Build history of the part. All positions in model axes, mm. Face numbers are marked on the shaded views. A direction names the side the tool comes from. Coordinates: 2 decimals unless noted, no trailing zeros. Order: outer loops, then holes, each group sorted by start corner. A loop starts at its lowest first (then second) coordinate and runs counter-clockwise, first axis right, second up. Notation, with made-up numbers: (9, 35) - (61, 35) arc R28 ccw to (61, 61) - close; hole circle Ø6 at (27.5, 33). An arc over 180 degrees is marked (long way). Return JSON: item names as keys, results as strings.
from build123d import *

# Parameters (mm, degrees)
EXTRUSION1_DEPTH = 70
EXTRUSION2_REACH = 3
ESQUISSE2_R      = 2
EXTRUSION3_REACH = 3
ESQUISSE3_R      = 2


with BuildPart() as part:
    # Esquisse1 → Extrusion1 (new body)
    with BuildSketch(Plane(origin=(0, 0, 0), x_dir=(1, 0, 0), z_dir=(0, 1, 0))):
        Polygon((0, 0), (0, 16), (1, 16), (1, 1), (16, 1), (16, 0), align=None)
    extrude(amount=EXTRUSION1_DEPTH)

    # Esquisse2 → Extrusion2 (cut, up to next)
    with BuildSketch(Plane(origin=(1, 0, 0), x_dir=(0, 0, -1), z_dir=(1, 0, 0)), mode=Mode.PRIVATE) as extrusion2_sk1:
        with Locations((8.5, 16.5)):
            Circle(ESQUISSE2_R)
    extrusion2_tool1 = extrude(extrusion2_sk1.sketch, amount=-EXTRUSION2_REACH, mode=Mode.PRIVATE) & part.part
    add(extrusion2_tool1.solids().sort_by_distance((1, 16.5, -8.5))[0], mode=Mode.SUBTRACT)
    # Esquisse2 → Extrusion2 (cut, up to next)
    with BuildSketch(Plane(origin=(1, 0, 0), x_dir=(0, 0, -1), z_dir=(1, 0, 0)), mode=Mode.PRIVATE) as extrusion2_sk2:
        with Locations((8.5, 6.5)):
            Circle(ESQUISSE2_R)
    extrusion2_tool2 = extrude(extrusion2_sk2.sketch, amount=-EXTRUSION2_REACH, mode=Mode.PRIVATE) & part.part
    add(extrusion2_tool2.solids().sort_by_distance((1, 6.5, -8.5))[0], mode=Mode.SUBTRACT)
    # Esquisse2 → Extrusion2 (cut, up to next)
    with BuildSketch(Plane(origin=(1, 0, 0), x_dir=(0, 0, -1), z_dir=(1, 0, 0)), mode=Mode.PRIVATE) as extrusion2_sk3:
        with Locations((8.5, 53.5)):
            Circle(ESQUISSE2_R)
    extrusion2_tool3 = extrude(extrusion2_sk3.sketch, amount=-EXTRUSION2_REACH, mode=Mode.PRIVATE) & part.part
    add(extrusion2_tool3.solids().sort_by_distance((1, 53.5, -8.5))[0], mode=Mode.SUBTRACT)
    # Esquisse2 → Extrusion2 (cut, up to next)
    with BuildSketch(Plane(origin=(1, 0, 0), x_dir=(0, 0, -1), z_dir=(1, 0, 0)), mode=Mode.PRIVATE) as extrusion2_sk4:
        with Locations((8.5, 63.5)):
            Circle(ESQUISSE2_R)
    extrusion2_tool4 = extrude(extrusion2_sk4.sketch, amount=-EXTRUSION2_REACH, mode=Mode.PRIVATE) & part.part
    add(extrusion2_tool4.solids().sort_by_distance((1, 63.5, -8.5))[0], mode=Mode.SUBTRACT)

    # Esquisse3 → Extrusion3 (cut, up to next)
    with BuildSketch(Plane(origin=(0, 0, -1), x_dir=(-1, 0, 0), z_dir=(0, 0, -1)), mode=Mode.PRIVATE) as extrusion3_sk1:
        with Locations((-8.5, 53.5)):
            Circle(ESQUISSE3_R)
    extrusion3_tool1 = extrude(extrusion3_sk1.sketch, amount=-EXTRUSION3_REACH, mode=Mode.PRIVATE) & part.part
    add(extrusion3_tool1.solids().sort_by_distance((8.5, 53.5, -1))[0], mode=Mode.SUBTRACT)
    # Esquisse3 → Extrusion3 (cut, up to next)
    with BuildSketch(Plane(origin=(0, 0, -1), x_dir=(-1, 0, 0), z_dir=(0, 0, -1)), mode=Mode.PRIVATE) as extrusion3_sk2:
        with Locations((-8.5, 63.5)):
            Circle(ESQUISSE3_R)
    extrusion3_tool2 = extrude(extrusion3_sk2.sketch, amount=-EXTRUSION3_REACH, mode=Mode.PRIVATE) & part.part
    add(extrusion3_tool2.solids().sort_by_distance((8.5, 63.5, -1))[0], mode=Mode.SUBTRACT)
    # Esquisse3 → Extrusion3 (cut, up to next)
    with BuildSketch(Plane(origin=(0, 0, -1), x_dir=(-1, 0, 0), z_dir=(0, 0, -1)), mode=Mode.PRIVATE) as extrusion3_sk3:
        with Locations((-8.5, 6.5)):
            Circle(ESQUISSE3_R)
    extrusion3_tool3 = extrude(extrusion3_sk3.sketch, amount=-EXTRUSION3_REACH, mode=Mode.PRIVATE) & part.part
    add(extrusion3_tool3.solids().sort_by_distance((8.5, 6.5, -1))[0], mode=Mode.SUBTRACT)
    # Esquisse3 → Extrusion3 (cut, up to next)
    with BuildSketch(Plane(origin=(0, 0, -1), x_dir=(-1, 0, 0), z_dir=(0, 0, -1)), mode=Mode.PRIVATE) as extrusion3_sk4:
        with Locations((-8.5, 16.5)):
            Circle(ESQUISSE3_R)
    extrusion3_tool4 = extrude(extrusion3_sk4.sketch, amount=-EXTRUSION3_REACH, mode=Mode.PRIVATE) & part.part
    add(extrusion3_tool4.solids().sort_by_distance((8.5, 16.5, -1))[0], mode=Mode.SUBTRACT)


solid = part.part
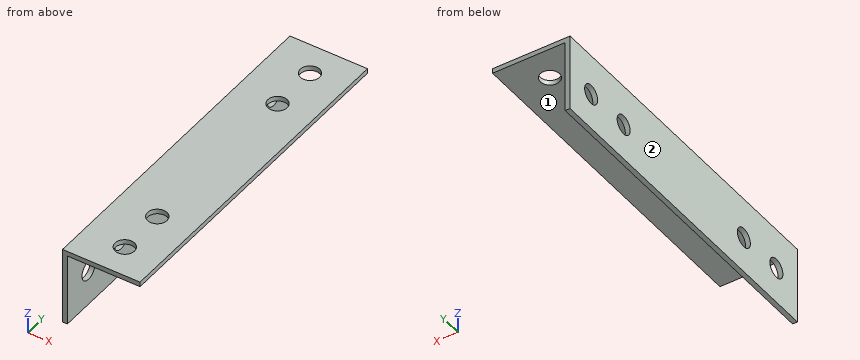
1. Cut at D-D on y = 19.5. Give the cut face in (x, z), plus the area to 3 significant figures.
Check values:
{"outline": "(0, -16) - (1, -16) - (1, -1) - (16, -1) - (16, 0) - (0, 0) - close", "area": "31.0 mm²"}
2. Cut at A-A on z = -8.5. Give the cut face in (x, y), plus the area to 3 significant figures.
Check values:
{"outline": "(0, 0) - (1, 0) - (1, 4.5) - (0, 4.5) - close; (0, 8.5) - (1, 8.5) - (1, 14.5) - (0, 14.5) - close; (0, 18.5) - (1, 18.5) - (1, 51.5) - (0, 51.5) - close; (0, 55.5) - (1, 55.5) - (1, 61.5) - (0, 61.5) - close; (0, 65.5) - (1, 65.5) - (1, 70) - (0, 70) - close", "area": "54.0 mm²"}
3. Drop flat-ended pins along their axis: pin 1 (6.5 mm diameter, centred on y = 53.5, z = -8.5, fed in from +X); pin 2 (1 mm diameter, centred on x = 11.5, y = 60, fed in from -Z). Give the stop position or say it passes through.
Check values:
{"pin 1": "x = 1", "pin 2": "z = -1"}
4. Cut at C-C on x = 8.5. Give the cut face in (y, z).
Check values:
{"outline": "(0, -1) - (4.5, -1) - (4.5, 0) - (0, 0) - close; (8.5, -1) - (14.5, -1) - (14.5, 0) - (8.5, 0) - close; (18.5, -1) - (51.5, -1) - (51.5, 0) - (18.5, 0) - close; (55.5, -1) - (61.5, -1) - (61.5, 0) - (55.5, 0) - close; (65.5, -1) - (70, -1) - (70, 0) - (65.5, 0) - close"}
5. Cut at B-B on y = 63.5. Give the cut face in (x, z), plus the area to 3 significant figures.
Check values:
{"outline": "(0, -16) - (1, -16) - (1, -10.5) - (0, -10.5) - close; (0, -6.5) - (1, -6.5) - (1, -1) - (6.5, -1) - (6.5, 0) - (0, 0) - close; (10.5, -1) - (16, -1) - (16, 0) - (10.5, 0) - close", "area": "23.0 mm²"}
6. Probe L1, parallel to Y at x = 0.85, z = -8.5; L2, parallel to Z at x = 12.25, y = 29.5; L3, parallel to X at y = 32.5, z = -2.75. List the from-to ranges inside material, lowest first.
Check values:
{"L1": "0 to 4.5, 8.5 to 14.5, 18.5 to 51.5, 55.5 to 61.5, 65.5 to 70", "L2": "-1 to 0", "L3": "0 to 1"}
7. Tool access for the marked faces 1 and 2: list every direction of +Z, -Z, +X, -X, +Y, -Y with a clear straight run to the whole face (end or side of a thin tool).
Check values:
{"face 1": "-Z, +X, +Y, -Y", "face 2": "+Z, -Z, -X, +Y, -Y"}
